Print and shaded views of the part. All mm, measured from the part's lowest x, y and z. Coordinates: 2 decimals unless noted, no trailing zeros. One line per question, with ' | ' between items. Start each with the question number.
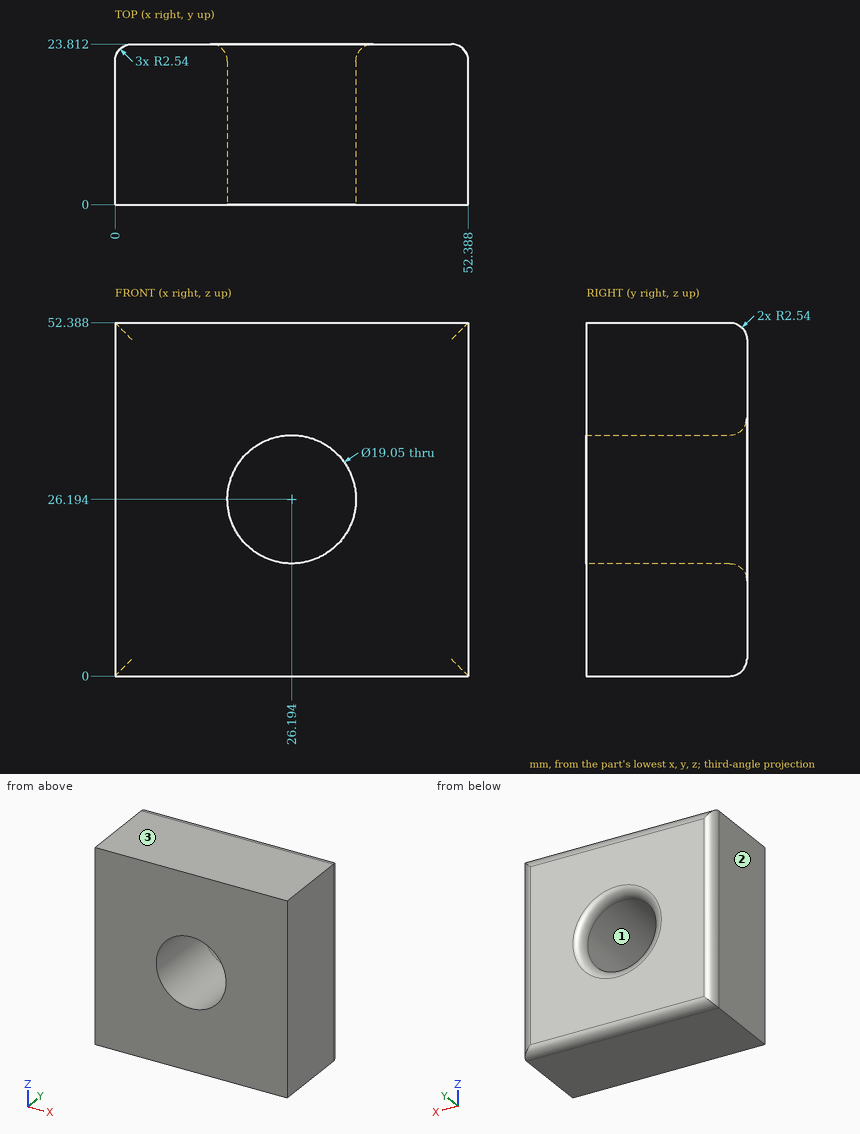
(1) Pin check, flat tip, straight feed: P1, Ø17, axis at x = 26.19, z = 26.19, coming from the -Y side. Stop position of the tip, or through.
(2) Drill centre lines: line 1 (X direction, y = 10.5, z = 18.5) (1 decimal); line 2 (X direction, y = 7.5, z = 21.5) (1 decimal); line 3 (Z direction, x = 19.5, y = 15) (1 decimal). Where is each one in solid material? Low to high. Write a range as [from, to].
(3) Two-plate mould, pull along Z, no slides. Class the marked faces 1, 2 and 3: pulls with the +Z half, pulls with the -Z half, needs draft (parallel to the pull), parting line crosses it, or undercut.
Computed values:
1) P1: through
2) line 1: [0, 20.6], [31.8, 52.4] | line 2: [0, 17.9], [34.5, 52.4] | line 3: [0, 19.4], [33, 52.4]
3) face 1: undercut | face 2: needs draft | face 3: pulls with the +Z half
